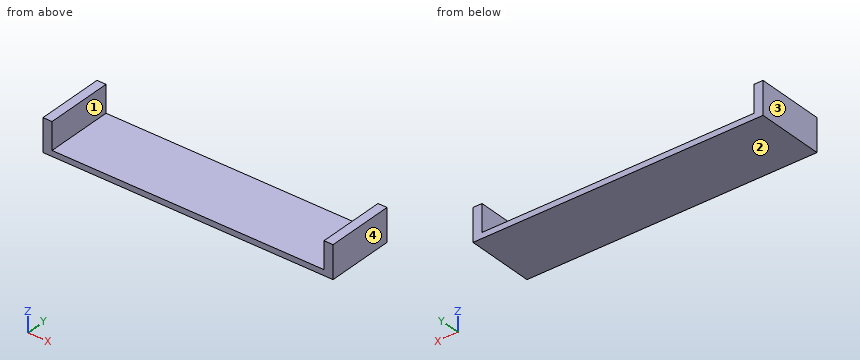
from build123d import *

# Parameters (mm, degrees)
SKETCH_2_W        = 8
SKETCH_2_H        = 60
EXTRUDE_1_DEPTH   = 24
EXTRUDE_1_2_DEPTH = 24
SKETCH_3_W        = 257
SKETCH_3_H        = 60
EXTRUDE_2_DEPTH   = 5


with BuildPart() as part:
    # Sketch 2 → Extrude 1 (new body)
    with BuildSketch(Plane.XY):
        with Locations((-19.51681736, 5.547854677)):
            Rectangle(SKETCH_2_W, SKETCH_2_H)
    extrude(amount=EXTRUDE_1_DEPTH)



with BuildPart() as body_2:
    # Sketch 2 → Extrude 1 2 (new body)
    with BuildSketch(Plane.XY):
        with Locations((229.48318264, 5.547854677)):
            Rectangle(SKETCH_2_W, SKETCH_2_H)
    extrude(amount=EXTRUDE_1_2_DEPTH)


with BuildPart() as part_1:
    add(part.part)

    add(body_2.part)  # Extrude 2 merges body 2
    # Sketch 3 → Extrude 2 (add)
    with BuildSketch(Plane(origin=(0, 0, 0), x_dir=(-1, 0, 0), z_dir=(0, 0, -1))):
        with Locations((-104.98318264, 5.547854677)):
            Rectangle(SKETCH_3_W, SKETCH_3_H)
    extrude(amount=EXTRUDE_2_DEPTH)


solid = part_1.part
Design review of the part built by this model. Coordinates are the model's own, in mm. Face numbers are marked on the shaded views. Round coordinates to 2 decimals unless told otherwise and drop trailing zeros. Write each loop counter-clockwise with the first axis right and the second up, starting at its lowest first coordinate (ties: lowest second). Pieces come first, ordered by that corner, then holes. Notation, with made-up numbers: (-6.75, 74) - (21.25, 74) arc R24 cw to (21.25, 101) - close; hole circle Ø5 at (-11, 40.25). An arc over 180 degrees is marked (long way). Return JSON: item names as keys, results as strings. Group by question number.
Item 1: Insertion check: P1, Ø10, axis at x = 153, y = 14, coming from the +Z side. The pin has a flat end and moves straight along its axis. Give the tip position at first contact, or say it passes through.
Item 2: We need section C-C on x = 26. Write out the cut boundary in (y, z), and give its area (3 significant figures).
Item 3: The part is to be moulded in two halves that separate along X. For the marked faces 1, 2, 3 and 4, say which applies: pulls with the +X half, pulls with the -X half, needs draft (parallel to the pull), parting line crosses it, or undercut.
Item 4: We need section B-B on y = 31.5. Write out the cut boundary in (x, z), and give its area (3 significant figures).
Item 5: For probe 1 along X at (y, z) = (8.5, 20.75); probe 2 along Z at (x, y) = (215.5, 22), list the stretches that pass through material, from the lowest coordinate up. Write a range as [from, to].
Item 6: We need section A-A on z = 16.25. Write out the cut boundary in (x, y).
Model answer:
{
 "1": {"P1": "stops at z = 0"},
 "2": {"outline": "(-24.45, -5) - (35.55, -5) - (35.55, 0) - (-24.45, 0) - close", "area": "300 mm²"},
 "3": {"face 1": "undercut", "face 2": "needs draft", "face 3": "pulls with the -X half", "face 4": "pulls with the +X half"},
 "4": {"outline": "(-23.52, -5) - (233.48, -5) - (233.48, 24) - (225.48, 24) - (225.48, 0) - (-15.52, 0) - (-15.52, 24) - (-23.52, 24) - close", "area": "1,670 mm²"},
 "5": {"probe 1": "x = [-23.52, -15.52], [225.48, 233.48]", "probe 2": "z = [-5, 0]"},
 "6": {"outline": "(-23.52, -24.45) - (-15.52, -24.45) - (-15.52, 35.55) - (-23.52, 35.55) - close; (225.48, -24.45) - (233.48, -24.45) - (233.48, 35.55) - (225.48, 35.55) - close"}
}
